Design review of the part built by this model. Coordinates are the model's own, in mm. Face numbers are marked on the shaded views. Give positions to 0.01 mm unless a question says otherwise; leave off trailing zeros. Write each loop counter-clockwise with the first axis right and the second up, starting at its lowest first coordinate (ties: lowest second). Pieces come first, ordered by that corner, then holes. Notation, with made-up numbers: (22.5, 65) -> (50.5, 65) arc R12 cw to (50.5, 88) -> close; hole circle Ø3 at (5, 84). An arc over 180 degrees is marked (long way). Write each question's results on one line, items separated by ' | '. Start each with the question number.
(1) To check wall thickness, follow probe 1 along X at (y, z) = (138.5, 3.25); probe 2 along Y at (x, z) = (33.5, 5.35); probe 3 along X at (y, z) = (190, 2.3). State the ranges of each line that lie inside material, in increasing order.
(2) Take a section at D-D (x = 14). State the section outline as (y, z) points.
(3) Mouldability with a two-part tool opening along Z and no side actions: class the marked faces 1 and 2 as released by +Z, released by -Z, zero draft, split by the parting line, or undercut.
(4) Take a section at C-C (x = 28). State the section outline as (y, z) points.
(5) Take a section at A-A (y = 121.5). State the section outline as (x, z) points, plus the area to 3 significant figures.
(6) Take a section at B-B (z = 2.65). State the section outline as (x, y) points.
(7) Clearance check with flat-ended pins moving along their axes: pin 1 (2 mm diameter, centred on x = 36, y = 177.5, fed in from -Z); pin 2 (1.8 mm diameter, centred on x = -32.5, z = 1.5, fed in from +Y); pin 3 (1.8 mm diameter, centred on x = -6.5, z = 3.5, fed in from -Y). State where each tip first meets the part, or that it passes through.
from build123d import *

# Parameters (mm, degrees)
BOSS_EXTRU_1_DEPTH      = 6
ENL_V_MAT_EXTRU_1_DEPTH = 10


with BuildPart() as part:
    # Esquisse1 → Boss.-Extru.1 (new body)
    with BuildSketch(Plane.XY):
        Polygon((-50, 0), (-50, 212), (-44, 212), (-44, 206), (-36, 206), (-36, 106), (-30, 106), (-30, 206), (-3, 206), (-3, 106), (3, 106), (3, 206), (30, 206), (30, 106), (36, 106), (36, 206), (44, 206), (44, 212), (50, 212), (50, 0), (44, 0), (44, 6), (-44, 6), (-44, 0), align=None)
    extrude(amount=BOSS_EXTRU_1_DEPTH)

    # Esquisse2 → Enlèv. mat.-Extru.1 (cut)
    with BuildSketch(Plane.XY.offset(6)):
        with BuildLine():
            Line((-44, 206), (44, 206))
            ThreePointArc((44, 206), (0, 184), (-44, 206))
        make_face()
    extrude(amount=-ENL_V_MAT_EXTRU_1_DEPTH, mode=Mode.SUBTRACT)


solid = part.part
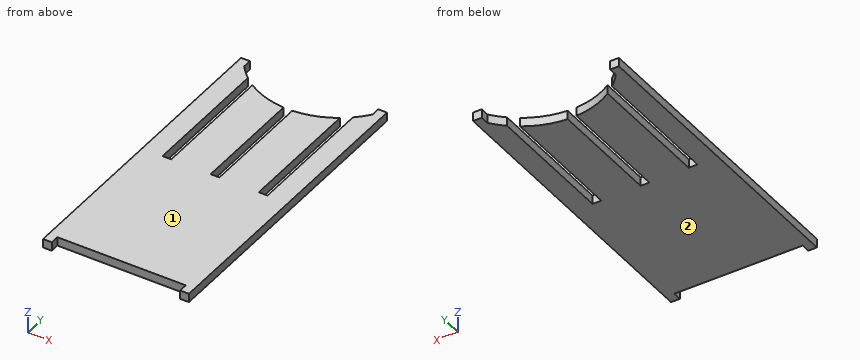
Report:
1) probe 1: -50 to -36, -30 to -3, 3 to 30, 36 to 50 | probe 2: 6 to 106 | probe 3: -50 to -36, -30 to -24.98, 24.98 to 30, 36 to 50
2) outline: (6, 0) -> (185.81, 0) -> (185.81, 6) -> (6, 6) -> close
3) face 1: released by +Z | face 2: released by -Z
4) outline: (6, 0) -> (191.66, 0) -> (191.66, 6) -> (6, 6) -> close
5) outline: (-50, 0) -> (-36, 0) -> (-36, 6) -> (-50, 6) -> close; (-30, 0) -> (-3, 0) -> (-3, 6) -> (-30, 6) -> close; (3, 0) -> (30, 0) -> (30, 6) -> (3, 6) -> close; (36, 0) -> (50, 0) -> (50, 6) -> (36, 6) -> close | area: 492 mm2
6) outline: (-50, 0) -> (-44, 0) -> (-44, 6) -> (44, 6) -> (44, 0) -> (50, 0) -> (50, 212) -> (44, 212) -> (44, 206) arc R55 cw to (36, 197.42) -> (36, 106) -> (30, 106) -> (30, 192.9) arc R55 cw to (3, 184.08) -> (3, 106) -> (-3, 106) -> (-3, 184.08) arc R55 cw to (-30, 192.9) -> (-30, 106) -> (-36, 106) -> (-36, 197.42) arc R55 cw to (-44, 206) -> (-44, 212) -> (-50, 212) -> close
7) pin 1: z = 0 | pin 2: y = 106 | pin 3: y = 6
